Read the model definition and answer for the solid it produces. Units are mm, in the model's axes. Face numbers are marked on the shaded views. Give positions to 0.01 mm unless a question says otherwise; leave off trailing zeros. Write each loop counter-clockwise with the first axis right and the second up, starting at its lowest first coordinate (ties: lowest second). Pieces come first, ordered by that corner, then holes. Notation, with made-up numbers: (28, -19) - (41, -19) arc R9 cw to (41, -11) - close; hole circle Ø5 at (31, -12). An arc over 180 degrees is marked (long way). Answer as CSV lines item,"result".
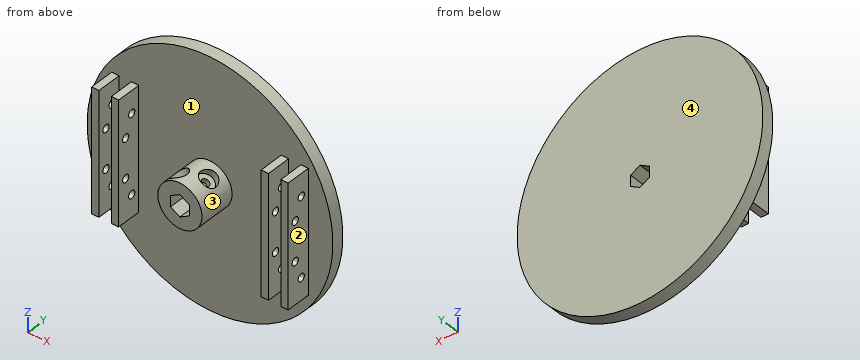
```python
from build123d import *

# Parameters (mm, degrees)
SKETCH2_R               = 9
BOSS_EXTRUDE1_DEPTH     = 20
CUT_EXTRUDE1_DEPTH      = 20
SKETCH4_R               = 50
SKETCH4_R_2             = 4.5
BOSS_EXTRUDE3_DEPTH     = 5
CUT_EXTRUDE2_DEPTH      = 9
CUT_EXTRUDE2_DEPTH_BACK = 9
SKETCH11_R              = 1.55
CUT_EXTRUDE9_DEPTH      = 9
CUT_EXTRUDE9_DEPTH_BACK = 9
SKETCH15_R              = 1.55
SKETCH16_W              = 3
SKETCH16_H              = 50
BOSS_EXTRUDE4_DEPTH     = 10
CUT_EXTRUDE10_REACH     = 106.881
SKETCH17_R              = 1.55
CUT_EXTRUDE11_START     = -11
SKETCH18_R              = 1.55
CUT_EXTRUDE11_DEPTH     = 11
CUT_EXTRUDE14_START     = 9
SKETCH19_R              = 3.5
CUT_EXTRUDE14_DEPTH     = 3
CUT_EXTRUDE15_START     = -6
SKETCH19_3_R            = 3.5
CUT_EXTRUDE15_DEPTH     = 3
CUT_EXTRUDE16_START     = 9
SKETCH20_R              = 3.5
CUT_EXTRUDE16_DEPTH     = 3
CUT_EXTRUDE17_START     = -6
SKETCH20_2_R            = 3.5
CUT_EXTRUDE17_DEPTH     = 3


with BuildPart() as part:
    # Sketch2 → Boss-Extrude1 (new body)
    with BuildSketch(Plane(origin=(0, 0, 0), x_dir=(1, 0, 0), z_dir=(0, 1, 0))):
        with Locations(Location((0, 0, 0), (0, 0, 270))):
            Circle(SKETCH2_R)
    extrude(amount=BOSS_EXTRUDE1_DEPTH)

    # Sketch3 → Cut-Extrude1 (cut)
    with BuildSketch(Plane(origin=(0, 20, 0), x_dir=(1, 0, 0), z_dir=(0, 1, 0))):
        Polygon((0, 4.4), (-3.810511777, 2.2), (-3.810511777, -2.2), (0, -4.4), (3.810511777, -2.2), (3.810511777, 2.2), align=None)
    extrude(amount=-CUT_EXTRUDE1_DEPTH, mode=Mode.SUBTRACT)

    # Sketch4 → Boss-Extrude3 (add)
    with BuildSketch(Plane(origin=(0, 20, 0), x_dir=(1, 0, 0), z_dir=(0, 1, 0))):
        with Locations(Location((0, 0, 0), (0, 0, 270))):
            Circle(SKETCH4_R)
        Circle(SKETCH4_R_2, mode=Mode.SUBTRACT)
    extrude(amount=-BOSS_EXTRUDE3_DEPTH)

    # Sketch11 → Cut-Extrude2 (cut, two sides: drawn at the far end of the back side and taken through both)
    with BuildSketch(Plane(origin=(0, 0, 0), x_dir=(-0.8660254037844387, 0, -0.49999999999999983), z_dir=(0.49999999999999983, 0, -0.8660254037844387)).offset(-CUT_EXTRUDE2_DEPTH_BACK)):
        with Locations(Location((0, 5, 0), (0, 0, 180))):
            Circle(SKETCH11_R)
    extrude(amount=CUT_EXTRUDE2_DEPTH + CUT_EXTRUDE2_DEPTH_BACK, mode=Mode.SUBTRACT)

    # Sketch15 → Cut-Extrude9 (cut, two sides: drawn at the far end of the back side and taken through both)
    with BuildSketch(Plane(origin=(0, 0, 0), x_dir=(-0.866025403784439, 0, 0.49999999999999944), z_dir=(-0.49999999999999944, 0, -0.866025403784439)).offset(-CUT_EXTRUDE9_DEPTH_BACK)):
        with Locations(Location((0, 9, 0), (0, 0, 270))):
            Circle(SKETCH15_R)
    extrude(amount=CUT_EXTRUDE9_DEPTH + CUT_EXTRUDE9_DEPTH_BACK, mode=Mode.SUBTRACT)

    # Sketch16 → Boss-Extrude4 (add)
    with BuildSketch(Plane.XZ.offset(-15)):
        with Locations((-30.5, 0)):
            Rectangle(SKETCH16_W, SKETCH16_H)
        with Locations((-38.5, 0)):
            Rectangle(SKETCH16_W, SKETCH16_H)
        with Locations((30.5, 0)):
            Rectangle(SKETCH16_W, SKETCH16_H)
        with Locations((38.5, 0)):
            Rectangle(SKETCH16_W, SKETCH16_H)
    extrude(amount=BOSS_EXTRUDE4_DEPTH)

    # Cut-Extrude10: up to this face of the body (flat: up to its plane)
    cut_extrude10_end = Plane(part.part.faces().sort_by_distance((-29, 10, 0))[0])
    # Sketch17 → Cut-Extrude10 (cut, up to the picked face)
    with BuildSketch(Plane.ZY.offset(40), mode=Mode.PRIVATE) as cut_extrude10_sk1:
        with Locations((-16, 11.5)):
            Circle(SKETCH17_R)
    cut_extrude10_tool1 = split(extrude(cut_extrude10_sk1.sketch, amount=-CUT_EXTRUDE10_REACH, mode=Mode.PRIVATE), bisect_by=cut_extrude10_end, keep=Keep.BOTH, mode=Mode.PRIVATE)
    # Sketch17 → Cut-Extrude10 (cut, up to the picked face)
    with BuildSketch(Plane.ZY.offset(40), mode=Mode.PRIVATE) as cut_extrude10_sk2:
        with Locations((-8, 8.5)):
            Circle(SKETCH17_R)
    cut_extrude10_tool2 = split(extrude(cut_extrude10_sk2.sketch, amount=-CUT_EXTRUDE10_REACH, mode=Mode.PRIVATE), bisect_by=cut_extrude10_end, keep=Keep.BOTH, mode=Mode.PRIVATE)
    # Sketch17 → Cut-Extrude10 (cut, up to the picked face)
    with BuildSketch(Plane.ZY.offset(40), mode=Mode.PRIVATE) as cut_extrude10_sk3:
        with Locations((8, 8.5)):
            Circle(SKETCH17_R)
    cut_extrude10_tool3 = split(extrude(cut_extrude10_sk3.sketch, amount=-CUT_EXTRUDE10_REACH, mode=Mode.PRIVATE), bisect_by=cut_extrude10_end, keep=Keep.BOTH, mode=Mode.PRIVATE)
    # Sketch17 → Cut-Extrude10 (cut, up to the picked face)
    with BuildSketch(Plane.ZY.offset(40), mode=Mode.PRIVATE) as cut_extrude10_sk4:
        with Locations((16, 11.5)):
            Circle(SKETCH17_R)
    cut_extrude10_tool4 = split(extrude(cut_extrude10_sk4.sketch, amount=-CUT_EXTRUDE10_REACH, mode=Mode.PRIVATE), bisect_by=cut_extrude10_end, keep=Keep.BOTH, mode=Mode.PRIVATE)
    add(cut_extrude10_tool1.solids().sort_by(Axis((-40, 11.5, -16), (1, 0, 0)))[0], mode=Mode.SUBTRACT)
    add(cut_extrude10_tool2.solids().sort_by(Axis((-40, 8.5, -8), (1, 0, 0)))[0], mode=Mode.SUBTRACT)
    add(cut_extrude10_tool3.solids().sort_by(Axis((-40, 8.5, 8), (1, 0, 0)))[0], mode=Mode.SUBTRACT)
    add(cut_extrude10_tool4.solids().sort_by(Axis((-40, 11.5, 16), (1, 0, 0)))[0], mode=Mode.SUBTRACT)

    # Sketch18 → Cut-Extrude11 (cut)
    with BuildSketch(Plane(origin=(40, 0, 0), x_dir=(0, 0, -1), z_dir=(1, 0, 0)).offset(CUT_EXTRUDE11_START)):
        with Locations(Location((-8, 8.5, 0), (0, 0, 180))):
            Circle(SKETCH18_R)
        with Locations(Location((8, 8.5, 0), (0, 0, 180))):
            Circle(SKETCH18_R)
        with Locations(Location((16, 11.5, 0), (0, 0, 180))):
            Circle(SKETCH18_R)
        with Locations(Location((-16, 11.5, 0), (0, 0, 180))):
            Circle(SKETCH18_R)
    extrude(amount=CUT_EXTRUDE11_DEPTH, mode=Mode.SUBTRACT)

    # Sketch19 → Cut-Extrude14 (cut)
    with BuildSketch(Plane(origin=(0, 0, 0), x_dir=(-0.866025403784439, 0, 0.49999999999999944), z_dir=(-0.49999999999999944, 0, -0.866025403784439)).offset(CUT_EXTRUDE14_START)):
        with Locations((0, 9)):
            Circle(SKETCH19_R)
    extrude(amount=-CUT_EXTRUDE14_DEPTH, mode=Mode.SUBTRACT)

    # Sketch19<3> → Cut-Extrude15 (cut)
    with BuildSketch(Plane(origin=(0, 0, 0), x_dir=(-0.866025403784439, 0, 0.49999999999999944), z_dir=(-0.49999999999999944, 0, -0.866025403784439)).offset(CUT_EXTRUDE15_START)):
        with Locations((0, 9)):
            Circle(SKETCH19_3_R)
    extrude(amount=-CUT_EXTRUDE15_DEPTH, mode=Mode.SUBTRACT)

    # Sketch20 → Cut-Extrude16 (cut)
    with BuildSketch(Plane(origin=(0, 0, 0), x_dir=(-0.8660254037844387, 0, -0.49999999999999983), z_dir=(0.49999999999999983, 0, -0.8660254037844387)).offset(CUT_EXTRUDE16_START)):
        with Locations((0, 5)):
            Circle(SKETCH20_R)
    extrude(amount=-CUT_EXTRUDE16_DEPTH, mode=Mode.SUBTRACT)

    # Sketch20<2> → Cut-Extrude17 (cut)
    with BuildSketch(Plane(origin=(0, 0, 0), x_dir=(-0.8660254037844387, 0, -0.49999999999999983), z_dir=(0.49999999999999983, 0, -0.8660254037844387)).offset(CUT_EXTRUDE17_START)):
        with Locations((0, 5)):
            Circle(SKETCH20_2_R)
    extrude(amount=-CUT_EXTRUDE17_DEPTH, mode=Mode.SUBTRACT)


solid = part.part
```
(1) Find the intervals of material crossed by L1, parallel to Z at x = 38.9, y = 8.5; L2, parallel to X at y = 13, z = -11.5; L3, parallel to Y at x = -38.8, z = -8, in increasing order.
Worked out:
L1,"z = -25 to -9.55, -6.45 to 6.45, 9.55 to 25"
L2,"x = -40 to -37, -32 to -29, 29 to 32, 37 to 40"
L3,"y = 5 to 6.95, 10.05 to 20"
(2) Each of these flat-tipped pins is pushed along its axis until it touches: P1, Ø10, axis at y = 5.5, z = 13, coming from the -X side; P2, Ø8, axis at y = 5, z = -8.5, coming from the +X side; P3, Ø1.9, axis at y = 8.5, z = -8, coming from the -X side; P4, Ø3, axis at x = -32, z = -38.5, coming from the +Y side. Where does it stop, or does it pass through?
Worked out:
P1,"stops at x = -40"
P2,"stops at x = 40"
P3,"stops at x = -1.21"
P4,"stops at y = 20"
(3) The mould has two halves that part along X. Classify the marked faces 1, 2, 3 and 4: +X half, -X half, draft (parallel to the pull), parting line (faces both ways), or undercut.
Worked out:
face 1,"undercut"
face 2,"+X half"
face 3,"undercut"
face 4,"draft"
(4) A cutting plane is placed at B-B (y = 18.5). Write down the section's boundary in (x, z), and give its area (3 significant figures).
Worked out:
outline,"circle Ø100 at (0, 0); hole (-3.81, -2.2) - (0, -4.4) - (3.81, -2.2) - (3.81, 2.2) - (0, 4.4) - (-3.81, 2.2) - close"
area,"7,800 mm^2"
(5) A cutting plane is placed at D-D (z = -16). Count the separate pieces of the cut face and the enclosed holes in it, and give its area (3 significant figures).
Worked out:
separate pieces,"5"
enclosed holes,"0"
area,"557 mm^2"
(6) A cutting plane is placed at C-C (x = 14). Write down the section's boundary in (y, z), and give its area (3 significant figures).
Worked out:
outline,"(15, -48) - (20, -48) - (20, 48) - (15, 48) - close"
area,"480 mm^2"
(7) A cutting plane is placed at A-A (z = 0). Write down the section's boundary in (x, y), and give its area (3 significant figures).
Worked out:
outline,"(-50, 15) - (-40, 15) - (-40, 5) - (-37, 5) - (-37, 15) - (-32, 15) - (-32, 5) - (-29, 5) - (-29, 15) - (-9, 15) - (-9, 0) - (-3.81, 0) - (-3.81, 20) - (-50, 20) - close; (3.81, 0) - (9, 0) - (9, 15) - (29, 15) - (29, 5) - (32, 5) - (32, 15) - (37, 15) - (37, 5) - (40, 5) - (40, 15) - (50, 15) - (50, 20) - (3.81, 20) - close"
area,"738 mm^2"
